```python
from build123d import *

# Parameters (mm, degrees)
SKETCH1_W           = 22.5
SKETCH1_H           = 22.7
BOSS_EXTRUDE1_DEPTH = 5.9
SKETCH2_W           = 4.7
SKETCH2_H           = 2.5
BOSS_EXTRUDE2_DEPTH = 11.8
CUT_EXTRUDE1_REACH  = 27.055
BOSS_EXTRUDE3_DEPTH = 4
SKETCH5_R           = 2.3
BOSS_EXTRUDE4_DEPTH = 3.2
SHELL3_START        = 1
SHELL3_OUTLINE_W    = 20.5
SHELL3_OUTLINE_H    = 9.8
SHELL3_DEPTH        = 20.7
SHELL3_START_2      = 21.7
SHELL3_2_DEPTH      = 4
SHELL3_START_3      = 16.9
SHELL3_3_DEPTH      = 0.5
SHELL3_START_4      = 25.7
SHELL3_4_OUTLINE_R  = 1.3
SHELL3_4_DEPTH      = 3.2


# Read off the part's stored shape, not the designer's step: Shell3
with BuildPart() as part:
    # Sketch1 → Boss-Extrude1 (new, symmetric)
    with BuildSketch(Plane.XY):
        with Locations((0, 11.35)):
            Rectangle(SKETCH1_W, SKETCH1_H)
    extrude(amount=BOSS_EXTRUDE1_DEPTH, both=True)

    # Sketch2 → Boss-Extrude2 (add)
    with BuildSketch(Plane.XY.offset(5.9)):
        with Locations((13.6, 17.15)):
            Rectangle(SKETCH2_W, SKETCH2_H)
    boss_extrude2 = extrude(amount=-BOSS_EXTRUDE2_DEPTH)

    # Sketch3 → Cut-Extrude1 (cut, up to next)
    with BuildSketch(Plane(origin=(0, 18.4, 0), x_dir=(1, 0, 0), z_dir=(0, 1, 0)), mode=Mode.PRIVATE) as cut_extrude1_sk1:
        with BuildLine():
            Line((15.95, 0.828555983), (14.409934208, 0.828555983))
            ThreePointArc((14.409934208, 0.828555983), (12.65, 0.178555983), (14.409934208, -0.471444017))
            Line((14.409934208, -0.471444017), (15.95, -0.471444017))
            Line((15.95, -0.471444017), (15.95, 0.828555983))
        make_face()
    cut_extrude1_tool1 = extrude(cut_extrude1_sk1.sketch, amount=-CUT_EXTRUDE1_REACH, mode=Mode.PRIVATE) & part.part
    cut_extrude1 = cut_extrude1_tool1.solids().sort_by_distance((14.234181, 18.4, -0.178556))[0]
    add(cut_extrude1, mode=Mode.SUBTRACT)

    # Mirror1: Boss-Extrude2, Cut-Extrude1 across plane
    add(boss_extrude2.mirror(Plane(origin=(0, 0, 0), x_dir=(0, 0, 1), z_dir=(1, 0, 0))))
    add(cut_extrude1.mirror(Plane(origin=(0, 0, 0), x_dir=(0, 0, 1), z_dir=(1, 0, 0))), mode=Mode.SUBTRACT)

    # Sketch4 → Boss-Extrude3 (add)
    with BuildSketch(Plane(origin=(0, 22.7, 0), x_dir=(1, 0, 0), z_dir=(0, 1, 0))):
        with BuildLine():
            Line((0, 2.487468593), (0.95, 2.5))
            ThreePointArc((0.95, 2.5), (3.45, 0), (0.95, -2.5))
            Line((0.95, -2.5), (-0.005844314, -2.5))
            ThreePointArc((-0.005844314, -2.5), (-11.249995949, 0.006913613), (0, 2.487468593))
        make_face()
    extrude(amount=BOSS_EXTRUDE3_DEPTH)

    # Sketch5 → Boss-Extrude4 (add)
    with BuildSketch(Plane(origin=(0, 26.7, 0), x_dir=(1, 0, 0), z_dir=(0, 1, 0))):
        with Locations(Location((-5.35, 0, 0), (0, 0, 270))):
            Circle(SKETCH5_R)
    extrude(amount=BOSS_EXTRUDE4_DEPTH)

    # Shell3 outline → Shell3 (cut)
    with BuildSketch(Plane(origin=(0, 0, 0), x_dir=(1, 0, 0), z_dir=(0, 1, 0)).offset(SHELL3_START)):
        Rectangle(SHELL3_OUTLINE_W, SHELL3_OUTLINE_H)
    extrude(amount=SHELL3_DEPTH, mode=Mode.SUBTRACT)

    # Shell3 2 outline → Shell3 2 (cut)
    with BuildSketch(Plane(origin=(0, 0, 0), x_dir=(1, 0, 0), z_dir=(0, 1, 0)).offset(SHELL3_START_2)):
        with BuildLine():
            Line((-0.685238484, -1.5), (0.95, -1.5))
            ThreePointArc((0.95, -1.5), (2.449997238, -0.002878764), (0.955757517, 1.49998895))
            Line((0.955757517, 1.49998895), (-0.67835846, 1.4784334))
            ThreePointArc((-0.67835846, 1.4784334), (-10.249986927, 0.01131871), (-0.685238484, -1.5))
        make_face()
    extrude(amount=SHELL3_2_DEPTH, mode=Mode.SUBTRACT)

    # Shell3 3 outline → Shell3 3 (cut)
    with BuildSketch(Plane(origin=(0, 0, 0), x_dir=(1, 0, 0), z_dir=(0, 1, 0)).offset(SHELL3_START_3)):
        with BuildLine():
            Line((-14.95, 4.9), (-14.95, 1.828555983))
            Line((-14.95, 1.828555983), (-14.780265456, 1.828555983))
            ThreePointArc((-14.780265456, 1.828555983), (-11.65, 0.178555983), (-14.780265456, -1.471444017))
            Line((-14.780265456, -1.471444017), (-14.95, -1.471444017))
            Line((-14.95, -1.471444017), (-14.95, -4.9))
            Line((-14.95, -4.9), (-10.25, -4.9))
            Line((-10.25, -4.9), (-10.25, 4.9))
            Line((-10.25, 4.9), (-14.95, 4.9))
        make_face()
        with BuildLine():
            Line((14.95, 4.9), (10.25, 4.9))
            Line((10.25, 4.9), (10.25, -4.9))
            Line((10.25, -4.9), (14.95, -4.9))
            Line((14.95, -4.9), (14.95, -1.471444017))
            Line((14.95, -1.471444017), (14.780265456, -1.471444017))
            ThreePointArc((14.780265456, -1.471444017), (11.65, 0.178555983), (14.780265456, 1.828555983))
            Line((14.780265456, 1.828555983), (14.95, 1.828555983))
            Line((14.95, 1.828555983), (14.95, 4.9))
        make_face()
    extrude(amount=SHELL3_3_DEPTH, mode=Mode.SUBTRACT)

    # Shell3 4 outline → Shell3 4 (cut)
    with BuildSketch(Plane(origin=(0, 0, 0), x_dir=(1, 0, 0), z_dir=(0, 1, 0)).offset(SHELL3_START_4)):
        with Locations((-5.35, 0)):
            Circle(SHELL3_4_OUTLINE_R)
    extrude(amount=SHELL3_4_DEPTH, mode=Mode.SUBTRACT)


solid = part.part
```
Read the model definition and answer for the solid it produces. Units are mm, in the model's axes. A direction names the side the tool comes from. Give positions to 0.01 mm unless a question says otherwise; leave off trailing zeros. Order: outer loops, then holes, each group sorted by start corner. A loop starts at its lowest first (then second) coordinate and runs counter-clockwise, first axis right, second up.
(1) Straight lines are drawn through the part: L1, parallel to Z at x = -13.65, y = 16.95; L2, parallel to Z at x = 1, y = 7.5; L3, parallel to X at y = 14, z = 1. For each, find the intervals that lie inside material, in ascending order.
(2) For faces 1 (the flat face through (-10, 22.7, 4)), 2 (the flat face through (12.5, 18.4, 0.1)), 3 (the flat face through (-10.25, 20, 0)), 4 (the flat face through (12.5, 15.9, 0.1)), determine the directions among +Z, -Z, +X, -X, +Y, -Y from which every point of the face is accessible in a straight line to the end or side of a thin tool.
(3) For a pull along Z with two mould halves and no side action, classify faces 5 (the cylindrical face through (3.45, 24.67, -0.05)), 6 (the cylindrical face through (-10.246, 23.672, -0.206)), 7 (the flat face through (0, 12, 5.9)), 8 (the cylindrical face through (-11.65, 17.15, -0.24)) as released by +Z, released by -Z, zero draft, split by the parting line, or undercut.
(4) Find section A-A (x = -13.65). Give the vertices of the cut face in (y, z).
(5) Find section B-B (y = 3.75). Give the vertices of the cut face in (x, z).
(6) Find section C-C (x = 6.5). Give the vertices of the cut face in (y, z).
(7) Given pin 1 (1.2 mm diameter, centred on x = 13.65, z = -0.18, fed in from -Y); pin 2 (2 mm diameter, centred on x = -5, z = -0.5, fed in from -Y); pin 3 (6 mm diameter, centred on y = 5, z = 4.5, fed in from +X); pin 4 (2.5 mm diameter, centred on x = 13, z = 0, fed in from -Y), each flat-ended and moving along its own axis, determine where each tip first touches the part or whether it passes through.
Result sheet:
1. L1: z = -5.9 to -4.9, -2.18 to -1.18, 0.82 to 1.82, 4.9 to 5.9
1. L2: z = -5.9 to -4.9, 4.9 to 5.9
1. L3: x = -11.25 to -10.25, 10.25 to 11.25
2. face 1: +Z, -X, +Y
2. face 2: +Z, -Z, +X, +Y
2. face 3: none
2. face 4: +Z, -Z, +X, -Y
3. face 5: split by the parting line
3. face 6: undercut
3. face 7: released by +Z
3. face 8: undercut
4. outline: (15.9, -5.9) - (18.4, -5.9) - (18.4, -1.18) - (15.9, -1.18) - close; (15.9, 0.82) - (18.4, 0.82) - (18.4, 5.9) - (15.9, 5.9) - close; hole (16.9, -4.9) - (17.4, -4.9) - (17.4, -2.18) - (16.9, -2.18) - close; hole (16.9, 1.82) - (17.4, 1.82) - (17.4, 4.9) - (16.9, 4.9) - close
5. outline: (-11.25, -5.9) - (11.25, -5.9) - (11.25, 5.9) - (-11.25, 5.9) - close; hole (-10.25, -4.9) - (10.25, -4.9) - (10.25, 4.9) - (-10.25, 4.9) - close
6. outline: (0, -5.9) - (22.7, -5.9) - (22.7, 5.9) - (0, 5.9) - close; hole (1, -4.9) - (21.7, -4.9) - (21.7, 4.9) - (1, 4.9) - close
7. pin 1: passes through
7. pin 2: stops at y = 0
7. pin 3: stops at x = 11.25
7. pin 4: stops at y = 15.9
